Here's the drawing with two shaded views (mm, measured from the low corner). I have some questions. A direction names the side the tool comes from. Coordinates: 2 decimals unless noted, no trailing zeros. Write each loop counter-clockwise with the first axis right and the second up, starting at its lowest first coordinate (ties: lowest second). Pieces come first, ordered by that corner, then holes. Notation, with made-up numbers: (-14.75, 52) -> (-8.75, 52) arc R18 ccw to (-8.75, 75) -> close; hole circle Ø7 at (45.25, 87.5). An arc over 180 degrees is marked (long way). Use one line per item in the form item = value.
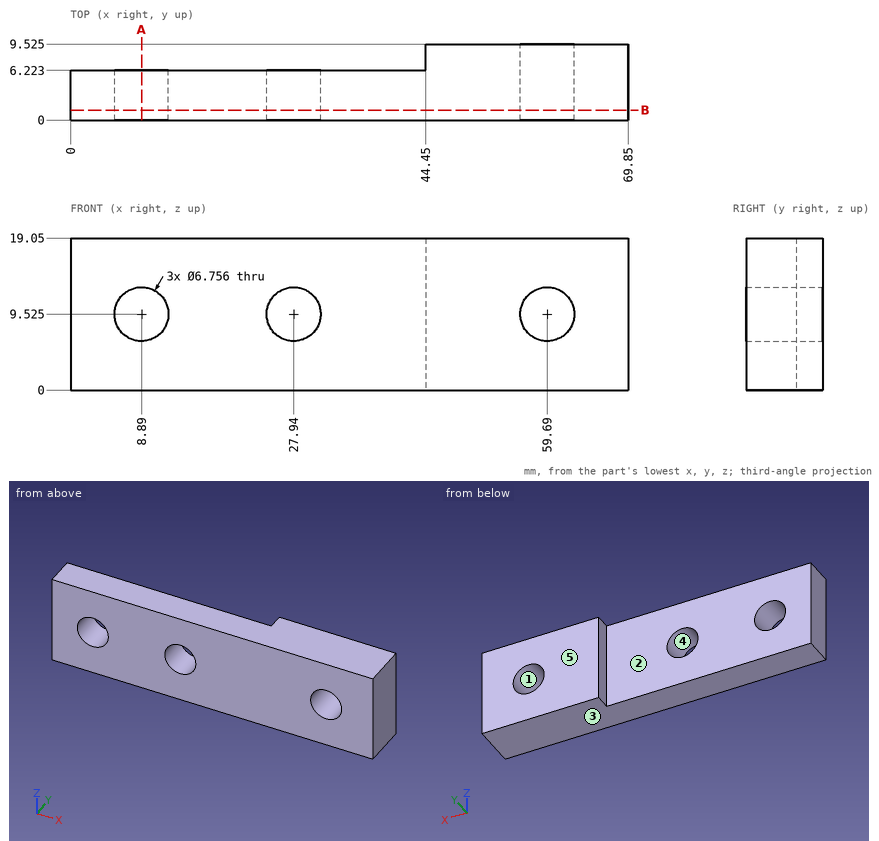
Q1. If I drill on line 1 (Z direction, x = 8.89, y = 4.75); line 2 (X direction, y = 1.25, z = 7.25); line 3 (Y direction, x = 17.5, z = 1.5), over which ranges is the centre line in solid material (lowest first)? Write a range as from..to.
Return value:
line_1 = 0..6.15, 12.9..19.05
line_2 = 0..6.39, 11.39..25.44, 30.44..57.19, 62.19..69.85
line_3 = 0..6.22
Q2. Suppose I cut it at A-A (x = 8.89). Write out the boundary of the cut face in (y, z).
Return value:
outline = (0, 0) -> (6.22, 0) -> (6.22, 6.15) -> (0, 6.15) -> close; (0, 12.9) -> (6.22, 12.9) -> (6.22, 19.05) -> (0, 19.05) -> close
Q3. Suppose I cut it at B-B (y = 1.25). Give the number of separate pieces and of enclosed holes in the cut face, then the cut area to 3 significant figures.
Return value:
separate_pieces = 1
enclosed_holes = 3
area = 1,220 mm2
Q4. Will this pin go through, and if not, where does the flat tip stop? pin 1 (9.5 mm diameter, centred on x = 32, z = 6.5, fed in from +Y).
Return value:
pin_1 = 6.22
Q5. Thinking about a two-plate mould opening in Z: for the marked faces 3, 4 and 5, which applies, released by +Z, released by -Z, zero draft, split by the parting line, or undercut?
Return value:
face_3 = released by -Z
face_4 = undercut
face_5 = zero draft
Q6. For the marked faces 1 and 2, which set-ups out of +Z, -Z, +X, -X, +Y, -Y let a thin tool reach every point of the face, with its end or its side?
Return value:
face_1 = +Y, -Y
face_2 = +Z, -Z, -X, +Y
